Autodesk Inventor part; units mm, degrees
ref_plane "YZ Plane" through (0, 0, 0) normal (1, 0, 0) x (0, 1, 0)
ref_plane "XZ Plane" through (0, 0, 0) normal (0, 1, 0) x (-1, 0, 0)
ref_plane "XY Plane" through (0, 0, 0) normal (0, 0, 1) x (1, 0, 0)
sketch "Sketch1" plane through (0, 0, 0) normal (0, 1, 0) x (-1, 0, 0)
  circle A0 centre (0, 0) radius 1.25
  circle A1 centre (0, 0) radius 7.5
  dimension "d0" = 2.5
  dimension "d1" = 15
extrude "Body" add sketch "Sketch1" along normal blind 2
chamfer "Bottom Chamfer" distance 1.5 distance2 4 1 edges at (7.5, 0, 0) measured on face at (-7.4757, 1.3333, -0.6035)
sketch "Sketch4" plane through (0, 0, 0) normal (1, 0, 0) x (0, 1, 0)
  line L0 (2, -7.5) -> (2, 7.5)
  line L1 (2, 3.35) -> (3, 3.35)
  line L2 (3, 3.35) -> (3, 3.65)
  line L3 (3, 3.65) -> (2, 3.65)
  line L4 (2, 3.65) -> (2, 3.35)
  line L5 (2, 3.65) -> (3, 3.55)
  line L6 (2, 3.65) -> (2.311367, 3.65) construction
  line L7 (3, 3.5) -> (2, 3.35)
  line L8 (-0.462273, 0) -> (2.77364, 0)
  point P0 (0, 0)
  point P1 (2, 0)
  point P2 (2, 3.65)
  dimension "d16" = 1
  dimension "d17" = 0.3
  dimension "d18" = 3.65
  dimension "d34" = 0.1
revolve "Centering Lip" add sketch "Sketch4" angle 360 about axis through (0, -10, 0) along (0, 1, 0) contours L0 L5 L2 L7
sketch "Sketch6" plane through (0, 0, 0) normal (0, 0, 1) x (1, 0, 0)
  line L0 (7.5, 2) -> (-7.5, 2)
  line L1 (7.5, 2) -> (7.2, 2)
  line L2 (7.2, 2) -> (7.2, 1.3)
  line L3 (7.2, 1.3) -> (7.5, 1.3)
  line L4 (7.5, 1.3) -> (7.5, 2)
  line L5 (-7.5, 1.5) -> (7.5, 1.5)
  line L6 (7.5, 1.3) -> (7.2, 1.5)
  line L7 (0, -0.4) -> (0, 2.4)
  point P0 (0, 0)
  dimension "d27" = 0.3
  dimension "d28" = 0.7
revolve "Revolution2" add sketch "Sketch6" angle 360 about axis through (0, -10, 0) along (0, 1, 0) contours L4 L6 L5
fillet "Fillet1" radius 0.3 2 edges at (0, 1.428, 7.308) (0, 1.428, -7.308)
sketch "Sketch7" plane through (0, 0, 0) normal (0, -1, 0) x (1, 0, 0)
  line L0 (-7.5, -0.1) -> (7.5, -0.1)
  line L1 (7.5, -0.1) -> (7.5, 7.5)
  line L2 (7.5, 7.5) -> (-7.5, 7.5)
  line L3 (-7.5, 7.5) -> (-7.5, -0.1)
  circle A0 centre (0, 0) radius 7.5
  point P0 (-7.499333, -0.1)
  point P1 (7.499333, -0.1)
  dimension "d31" = 0.1
sketch "Sketch7 outline for Extrusion5" plane through (0, 0, 0) normal (0, -1, 0) x (1, 0, 0)
  arc A0 (7.499333, -0.1) -> (-7.499333, -0.1) centre (0, 0) ccw
  line L0 (-7.499333, -0.1) -> (7.499333, -0.1)
extrude "Extrusion5" cut sketch "Sketch7 outline for Extrusion5" against normal through all
chamfer "Chamfer3" distance 0.2 angle 45 1 edges at (0, 2, -3.65)
properties part number "Wire Passthrough Resin Seal"
CAD build for the part. Positions are in the model's coordinates, mm. A direction names the side the tool comes from. Coordinates: 2 decimals unless noted, no trailing zeros. Write each loop counter-clockwise with the first axis right and the second up, starting at its lowest first coordinate (ties: lowest second). Pieces come first, ordered by that corner, then holes.
(1) Drill centre lines: probe 1 along Y at (x, z) = (-5, -5.5); probe 2 along Y at (x, z) = (-2, -0.5); probe 3 along Z at (x, y) = (0.25, 1.55). Where is each one in solid material? Low to high.
(2) Cut at C-C, the plane y = 2.4. List the corners of the cut face in (x, z), and give its area (3 significant figures).
(3) 3-axis set-ups, long thin cutter, end or side, ignore diameter. For faces 4 (the face through (0, 2, -5)), 5 (the face through (0, 2, -2)), 6 (the face through (4, 1, -0.1)): which of +Z, -Z, +X, -X, +Y, -Y reach the whole face in a straight line?
(4) Two-plate mould, pull along X, no slides. Class faces 1 (the face through (-0.08, 2.59, -3.59)), 2 (the face through (-4, 1, -0.1)), 3 (the face through (-0.03, 0.99, -1.25)): +X half, -X half, draft (parallel to the pull), parting line (faces both ways), or undercut.
(5) Cut at A-A, the plane x = 0. List the corners of the cut face in (y, z), and give its area (3 significant figures).
(6) Flat gauge pin, fed straight in: pin 1 (2.5 mm diameter, centred on x = 0.5, z = -1.5, fed in from +Y). Where does the tip first touch, or does it go through?
Geometry says:
1. probe 1: y = 1.34 to 2
1. probe 2: y = 0 to 2
1. probe 3: z = -7.5 to -1.22
2. outline: (-3.61, -0.1) arc R3.61 ccw to (3.61, -0.1) - (3.41, -0.1) arc R3.41 cw to (-3.41, -0.1) - close
2. area: 2.17 mm2
3. face 4: -Z, +Y
3. face 5: +Z, +Y
3. face 6: +Z, +X, -X, +Y, -Y
4. face 1: parting line
4. face 2: draft
4. face 3: undercut
5. outline: (0, -3.5) - (1.37, -7.16) arc R0.3 cw to (1.34, -7.44) - (1.3, -7.5) - (2, -7.5) - (2, -3.85) - (2.2, -3.63) - (3, -3.55) - (3, -3.5) - (2, -3.35) - (2, -1.25) - (0, -1.25) - close
5. area: 9.72 mm2
6. pin 1: stops at y = 2
